Print and shaded views of the part. All mm, measured from the part's lowest x, y and z. A direction names the side the tool comes from. Round coordinates to 2 decimals unless told otherwise and drop trailing zeros. Order: outer loops, then holes, each group sorted by start corner. A loop starts at its lowest first (then second) coordinate and runs counter-clockwise, first axis right, second up. Notation, with made-up numbers: M 79,-36 L 118,-36 A21 ccw 118,-26 Z; hole C 38,69 d11. An arc over 180 degrees is marked long. Write each question's results on one line, items separated by ' | '. Start each with the question number.
1. Which spindle directions (+Z, -Z, +X, -X, +Y, -Y) get a long thin tool onto all of the face, cutting with end or side? Do the marked faces 4 and 5. Say none if no direction does.
2. Band-saw the part on C-C, the plane y = 10. List the corners of the cut face in (x, z).
3. Drop flat-ended pins along their axis: pin 1 Ø1 at (y, z) = (2.5, 2) entering from -X; pin 2 Ø3.5 at (x, z) = (10, 6) entering from +Y. Give the stop position or say it passes through.
4. Two-plate mould, pull along X, no slides. Class the marked faces 1, 2 and 3: +X half, -X half, draft (parallel to the pull), parting line (faces both ways), or undercut.
5. Band-saw the part on D-D, the plane x = 16. List the corners of the cut face in (y, z).
6. Probe L1, parallel to X at y = 8.25, z = 11.5; L2, parallel to Z at x = 12.5, y = 5; L3, parallel to Y at x = 8.5, z = 3. List the from-to ranges inside material, lowest first. Write a range as [from, to].
7. Band-saw the part on A-A, the plane z = 8. List the corners of the cut face in (x, y).
8. Band-saw the part on B-B, the plane x = 11.25. List the corners of the cut face in (y, z).
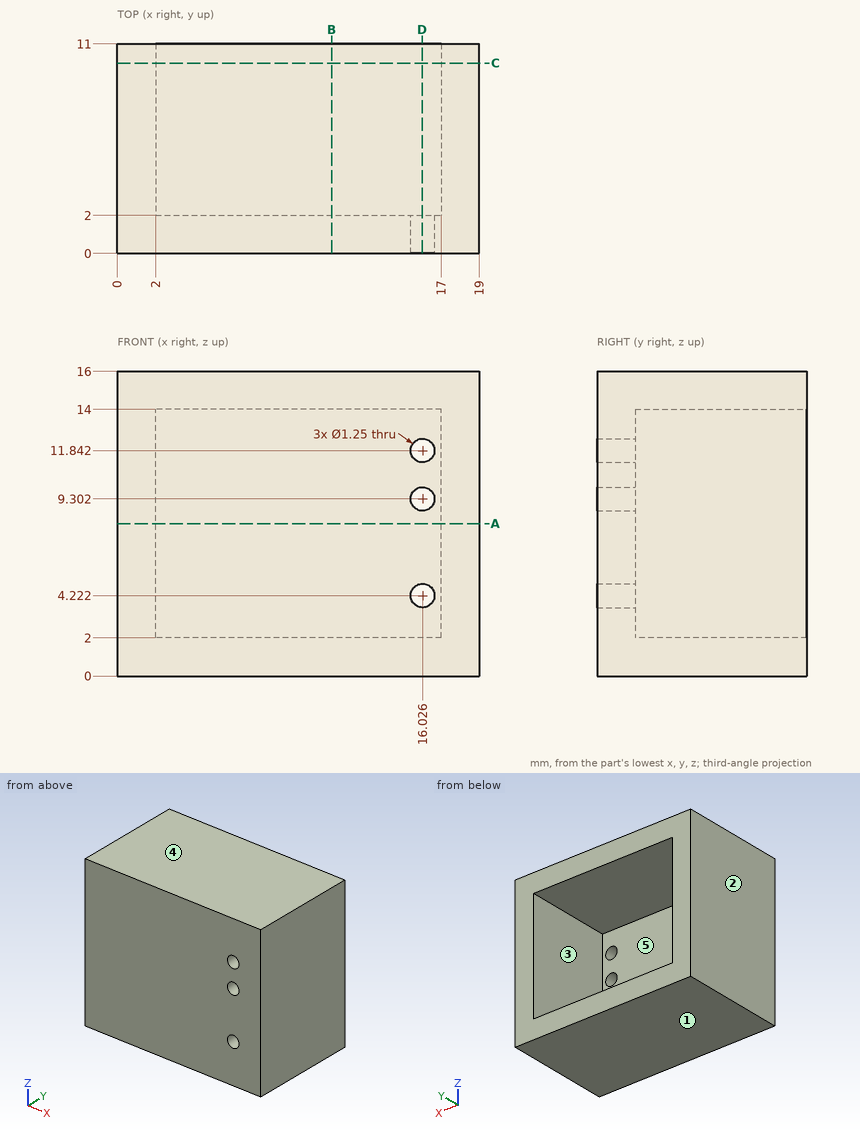
Solution:
1) face 4: +Z, +X, -X, +Y, -Y | face 5: +Y
2) outline: M 0,0 L 19,0 L 19,16 L 0,16 Z; hole M 2,2 L 17,2 L 17,14 L 2,14 Z
3) pin 1: x = 0 | pin 2: y = 2
4) face 1: draft | face 2: -X half | face 3: undercut
5) outline: M 0,0 L 11,0 L 11,2 L 2,2 L 2,3.6 L 0,3.6 Z; M 0,4.85 L 2,4.85 L 2,8.68 L 0,8.68 Z; M 0,9.93 L 2,9.93 L 2,11.22 L 0,11.22 Z; M 0,12.47 L 2,12.47 L 2,14 L 11,14 L 11,16 L 0,16 Z
6) L1: [0, 2], [17, 19] | L2: [0, 2], [14, 16] | L3: [0, 2]
7) outline: M 0,0 L 19,0 L 19,11 L 17,11 L 17,2 L 2,2 L 2,11 L 0,11 Z
8) outline: M 0,0 L 11,0 L 11,2 L 2,2 L 2,14 L 11,14 L 11,16 L 0,16 Z
